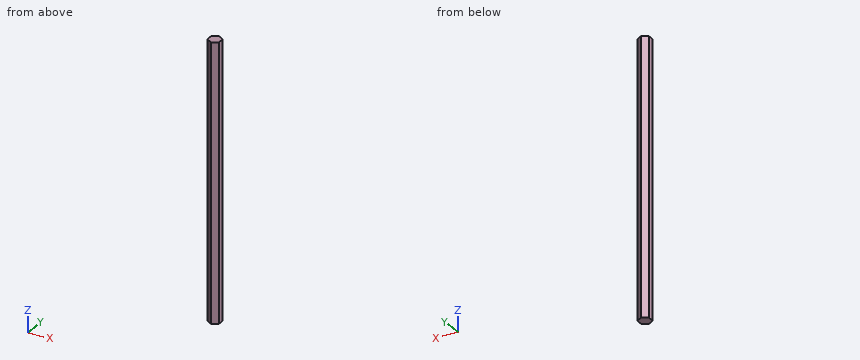
```python
from build123d import *

# Parameters (mm, degrees)
BOSS_EXTRUDE1_DEPTH = 152.4


with BuildPart() as part:
    # Sketch3 → Boss-Extrude1 (new, symmetric)
    with BuildSketch(Plane.XY):
        Polygon((0, 7.332348419), (6.35, 3.666174209), (6.35, -3.666174209), (0, -7.332348419), (-6.35, -3.666174209), (-6.35, 3.666174209), align=None)
    extrude(amount=BOSS_EXTRUDE1_DEPTH, both=True)


solid = part.part
```
Input: part model. Units: mm. Frame: model coordinates. Give positions to 0.01 mm unless a question says otherwise; leave off trailing zeros. Order: outer loops, then holes, each group sorted by start corner. A loop starts at its lowest first (then second) coordinate and runs counter-clockwise, first axis right, second up. Notation, with made-up numbers: M 89,31 L 141,31 A21 cw 141,64 Z; hole C 77,79.5 d3. An arc over 180 degrees is marked long. Return JSON: item names as keys, results as strings.
1) Contact query for flat-ended pins moving along their axis: pin 1 (1 mm diameter, centred on x = 1, z = 18.5, fed in from +Y); pin 2 (6 mm diameter, centred on x = 5, z = 121.5, fed in from -Y); pin 3 (1.5 mm diameter, centred on x = -4, z = -72, fed in from +Y). Output: stop coordinate, or through.
Taken from the geometry:
{"pin 1": "stops at y = 7.04", "pin 2": "stops at y = -6.18", "pin 3": "stops at y = 5.46"}
2) Line query: L1, parallel to Y at x = 0.25, z = -90.5; L2, parallel to Y at x = 3, z = 23.5; L3, parallel to X at y = -4.5, z = -131. Output: solid intervals per line, ascending. Write a range as [from, to].
Taken from the geometry:
{"L1": "y = [-7.19, 7.19]", "L2": "y = [-5.6, 5.6]", "L3": "x = [-4.91, 4.91]"}
3) Section query B-B on x = 4. Output: boundary loops of the cut face in (y, z), and give its area (3 significant figures).
Taken from the geometry:
{"outline": "M -5.02,-152.4 L 5.02,-152.4 L 5.02,152.4 L -5.02,152.4 Z", "area": "3,060 mm2"}
4) Section query A-A on z = 20. Output: boundary loops of the cut face in (x, y).
Taken from the geometry:
{"outline": "M -6.35,-3.67 L 0,-7.33 L 6.35,-3.67 L 6.35,3.67 L 0,7.33 L -6.35,3.67 Z"}
